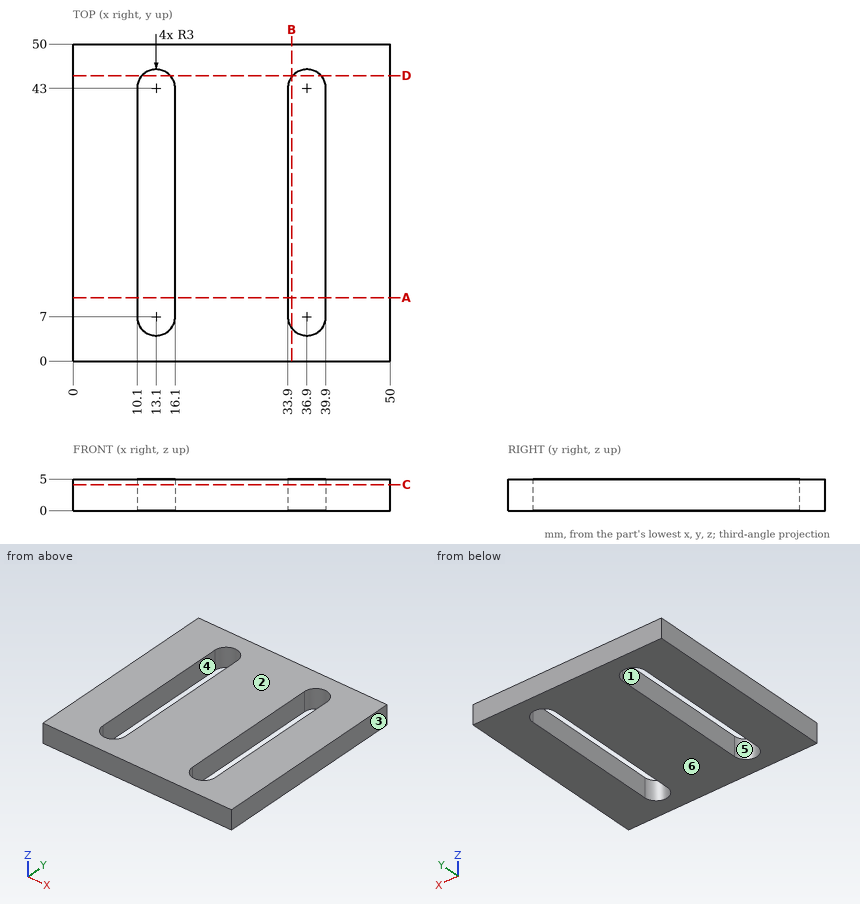
Verification items for this drawing (mm, ordinates from the low corner). A direction names the side the tool comes from. Coordinates: 2 decimals unless noted, no trailing zeros. Order: outer loops, then holes, each group sorted by start corner. A loop starts at its lowest first (then second) coordinate and runs counter-clockwise, first axis right, second up. Notation, with made-up numbers: M 1,-24 L 53,-24 A21 ccw 53,-15 Z; hole C 81,13 d5. An arc over 180 degrees is marked long. One line per item, written item: value. Start each with the question number.
Item 1: Access from +Z, -Z, +X, -X, +Y, -Y to the whole of each face (thin tool, end or side, straight path). Record for the marked faces 5 and 6.
Item 2: Thickness scan on probe 1 along X at (y, z) = (12, 1.9); probe 2 along X at (y, z) = (4.5, 4.15); probe 3 along Y at (x, z) = (36, 4.2). Record the ranges inside material, lowest first.
Item 3: Mould release check, pull along X, two halves, no side actions. Record for the marked faces 1, 2, 3 and 4: pulls with the +X half, pulls with the -X half, needs draft (parallel to the pull), parting line crosses it, or undercut.
Item 4: Sectioned sample at C-C on z = 4.1. Record the cut outline in (x, y).
Item 5: Sectioned sample at A-A on y = 10. Record the cut outline in (x, z), then the cut area to 3 significant figures.
Item 6: Sectioned sample at D-D on y = 45. Record the cut outline in (x, z).
Item 7: Sectioned sample at B-B on x = 34.5. Record the cut outline in (y, z), then the cut area to 3 significant figures.
Calculated:
1. face 5: +Z, -Z
1. face 6: -Z, +X, -X, +Y, -Y
2. probe 1: 0 to 10.1, 16.1 to 33.9, 39.9 to 50
2. probe 2: 0 to 11.44, 14.76 to 35.24, 38.56 to 50
2. probe 3: 0 to 4.14, 45.86 to 50
3. face 1: undercut
3. face 2: needs draft
3. face 3: pulls with the +X half
3. face 4: undercut
4. outline: M 0,0 L 50,0 L 50,50 L 0,50 Z; hole M 10.1,7 A3 ccw 16.1,7 L 16.1,43 A3 ccw 10.1,43 Z; hole M 33.9,7 A3 ccw 39.9,7 L 39.9,43 A3 ccw 33.9,43 Z
5. outline: M 0,0 L 10.1,0 L 10.1,5 L 0,5 Z; M 16.1,0 L 33.9,0 L 33.9,5 L 16.1,5 Z; M 39.9,0 L 50,0 L 50,5 L 39.9,5 Z
5. area: 190 mm^2
6. outline: M 0,0 L 10.86,0 L 10.86,5 L 0,5 Z; M 15.34,0 L 34.66,0 L 34.66,5 L 15.34,5 Z; M 39.14,0 L 50,0 L 50,5 L 39.14,5 Z
7. outline: M 0,0 L 5.2,0 L 5.2,5 L 0,5 Z; M 44.8,0 L 50,0 L 50,5 L 44.8,5 Z
7. area: 52.0 mm^2
